Could you check a few things on this model? Use its own coordinates, in mm. Face numbers are marked on the shaded views. Round coordinates to 2 decimals unless told otherwise and drop trailing zeros. Loops run counter-clockwise (first coordinate to the right, second up) from the corner with the lowest first, then second, coordinate; pieces in that order, holes last. Notation, with made-up numbers: (63, -27.75) -> (75, -27.75) arc R26 ccw to (75, 7.25) -> close; hole circle Ø11 at (63.5, 53). An arc over 180 degrees is marked (long way). One line per item, written item: value.
```python
from build123d import *

# Parameters (mm, degrees)
SKIZZE2_W                       = 28
SKIZZE2_H                       = 28
SKIZZE2_R                       = 1.5
AUFSATZ_LINEAR_AUSTRAGEN1_DEPTH = 40
SKIZZE3_W                       = 24
SKIZZE3_H                       = 5
SCHNITT_LINEAR_AUSTRAGEN1_DEPTH = 30
F_4_0_4_DURCHMESSER_BOHRUNG1_D  = 4
VERRUNDUNG1_R                   = 2


with BuildPart() as part:
    # Skizze2 → Aufsatz-Linear austragen1 (new body)
    with BuildSketch(Plane(origin=(0, 0, 0), x_dir=(1, 0, 0), z_dir=(0, 1, 0))):
        with Locations((-10.243240712, -0.002346974)):
            Rectangle(SKIZZE2_W, SKIZZE2_H)
        with Locations(Location((-20.243240712, 9.997653026, 0), (0, 0, 270))):
            Circle(SKIZZE2_R, mode=Mode.SUBTRACT)
        with Locations(Location((-0.243240712, 9.997653026, 0), (0, 0, 270))):
            Circle(SKIZZE2_R, mode=Mode.SUBTRACT)
        with Locations(Location((-20.243240712, -10.002346974, 0), (0, 0, 270))):
            Circle(SKIZZE2_R, mode=Mode.SUBTRACT)
        with Locations(Location((-0.243240712, -10.002346974, 0), (0, 0, 270))):
            Circle(SKIZZE2_R, mode=Mode.SUBTRACT)
    extrude(amount=AUFSATZ_LINEAR_AUSTRAGEN1_DEPTH)

    # Skizze3 → Schnitt-Linear austragen1 (cut)
    with BuildSketch(Plane(origin=(0, 40, 0), x_dir=(1, 0, 0), z_dir=(0, 1, 0))):
        with Locations((-12.243240712, -0.002346974)):
            Rectangle(SKIZZE3_W, SKIZZE3_H)
    extrude(amount=-SCHNITT_LINEAR_AUSTRAGEN1_DEPTH, mode=Mode.SUBTRACT)

    # Ø4.0 (4) Durchmesser Bohrung1 (through all)
    with Locations(Plane.XY.offset(14.002346974)):
        with Locations((-10.243240712, 15.5), (-10.243240712, 35.5), (-10.243240712, 25.5)):
            Hole(F_4_0_4_DURCHMESSER_BOHRUNG1_D / 2)

    # Verrundung1
    verrundung1_edges = [part.edges().sort_by_distance(p)[0] for p in [
        (3.756759288, 40, 0.002346974),
        (-10.243240712, 40, -13.997653026),
        (-12.243240712, 40, 2.502346974),
        (-0.243240712, 40, 0.002346974),
        (-12.243240712, 40, -2.497653026),
        (-10.243240712, 40, 14.002346974),
    ]]
    fillet(verrundung1_edges, radius=VERRUNDUNG1_R - 0.0001)  # a hair under: the kernel refuses the full size


solid = part.part
```
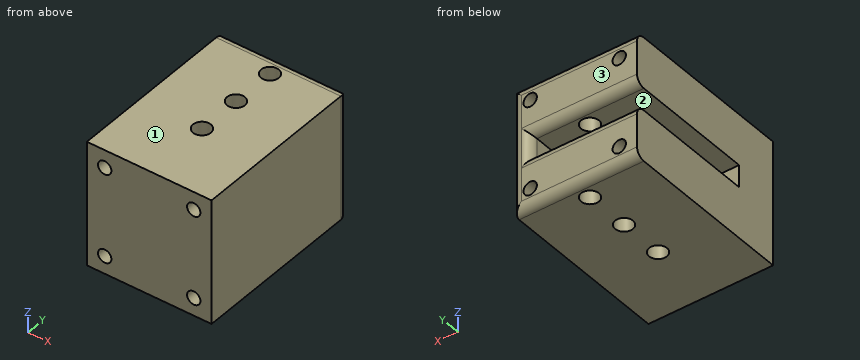
(1) Please list where these lines run through material, in increasing order: L1, parallel to Y at x = -10.25, z = -6.5; L2, parallel to Y at x = -10.25, z = 4; L3, parallel to Z at x = -15.25, y = 30.
Results below:
L1: y = 0 to 13.5, 17.5 to 23.5, 27.5 to 33.5, 37.5 to 40
L2: y = 0 to 13.5, 17.5 to 23.5, 27.5 to 33.5, 37.5 to 39.94
L3: z = -14 to -2.5, 2.5 to 14
(2) Imagine slicing it at C-C on z = 6. Write out the boundary of the cut face in (x, y), then the cut area to 3 significant figures.
Results below:
outline: (-24.24, 0) -> (3.76, 0) -> (3.76, 38) arc R2 ccw to (1.76, 40) -> (-24.24, 40) -> close; hole circle Ø4 at (-10.24, 15.5); hole circle Ø4 at (-10.24, 25.5); hole circle Ø4 at (-10.24, 35.5)
area: 1,080 mm²
(3) Imagine slicing it at A-A on z = 9.25. Write out the boundary of the cut face in (x, y), then the cut area to 3 significant figures.
Results below:
outline: (-24.24, 0) -> (-21.54, 0) -> (-21.54, 40) -> (-24.24, 40) -> close; (-18.95, 0) -> (-1.54, 0) -> (-1.54, 40) -> (-18.95, 40) -> close; (1.05, 0) -> (3.76, 0) -> (3.76, 38) arc R2 ccw to (1.76, 40) -> (1.05, 40) -> close; hole circle Ø4 at (-10.24, 15.5); hole circle Ø4 at (-10.24, 25.5); hole circle Ø4 at (-10.24, 35.5)
area: 874 mm²
(4) We'd pull the mould along Z, two halves only. Please class the marked faces 1, 2 and 3: +Z half, -Z half, draft (parallel to the pull), parting line (faces both ways), or undercut.
Results below:
face 1: +Z half
face 2: undercut
face 3: draft
(5) Imagine slicing it at B-B on y = 15.5. Write out the boundary of the cut face in (x, z), then the cut area to 3 significant figures.
Results below:
outline: (-24.24, -14) -> (-12.24, -14) -> (-12.24, -2.5) -> (-24.24, -2.5) -> close; (-24.24, 2.5) -> (-12.24, 2.5) -> (-12.24, 14) -> (-24.24, 14) -> close; (-8.24, -14) -> (3.76, -14) -> (3.76, 14) -> (-8.24, 14) -> (-8.24, 2.5) -> (-0.24, 2.5) -> (-0.24, -2.5) -> (-8.24, -2.5) -> close; hole circle Ø3 at (-20.24, -10); hole circle Ø3 at (-20.24, 10); hole circle Ø3 at (-0.24, -10); hole circle Ø3 at (-0.24, 10)
area: 544 mm²
(6) For pin 1 Ø3 at (x, y) = (-10.24, 35.5) entering from +Z; pin 2 Ø4 at (x, z) = (-13, -1) entering from +Y; pin 3 Ø1.5 at (x, z) = (-11, -1.5) entering from +Y, each with a flat end and sliding along its axis, tell me the tip position at first contact or that it passes through.
Results below:
pin 1: passes through
pin 2: stops at y = 39.33
pin 3: stops at y = 10
